Build history of the part. All positions in model axes, mm. Face numbers are marked on the shaded views. Give positions to 0.01 mm unless a question says otherwise; leave off trailing zeros. Order: outer loops, then holes, each group sorted by start corner. A loop starts at its lowest first (then second) coordinate and runs counter-clockwise, first axis right, second up. Notation, with made-up numbers: M -17.75,-26.5 L -13.75,-26.5 A15 ccw -13.75,1.5 Z; hole C 70.25,-22.5 d2. An arc over 180 degrees is marked long. Answer as CSV lines item,"result".
from build123d import *

# Parameters (mm, degrees)
CROQUIS1_W              = 120
CROQUIS1_H              = 120
CROQUIS1_R              = 3
CROQUIS1_W_2            = 80
CROQUIS1_H_2            = 80
SALIENTE_EXTRUIR1_DEPTH = 2.7


with BuildPart() as part:
    # Croquis1 → Saliente-Extruir1 (new body)
    with BuildSketch(Plane.XY):
        Rectangle(CROQUIS1_W, CROQUIS1_H)
        with Locations(Location((-40, 50, 0), (0, 0, 180))):
            Circle(CROQUIS1_R, mode=Mode.SUBTRACT)
        with Locations(Location((0, 50, 0), (0, 0, 180))):
            Circle(CROQUIS1_R, mode=Mode.SUBTRACT)
        with Locations(Location((40, 50, 0), (0, 0, 180))):
            Circle(CROQUIS1_R, mode=Mode.SUBTRACT)
        with Locations(Location((-40, -50, 0), (0, 0, 180))):
            Circle(CROQUIS1_R, mode=Mode.SUBTRACT)
        with Locations(Location((0, -50, 0), (0, 0, 180))):
            Circle(CROQUIS1_R, mode=Mode.SUBTRACT)
        with Locations(Location((40, -50, 0), (0, 0, 180))):
            Circle(CROQUIS1_R, mode=Mode.SUBTRACT)
        Rectangle(CROQUIS1_W_2, CROQUIS1_H_2, mode=Mode.SUBTRACT)
    extrude(amount=SALIENTE_EXTRUIR1_DEPTH)


solid = part.part
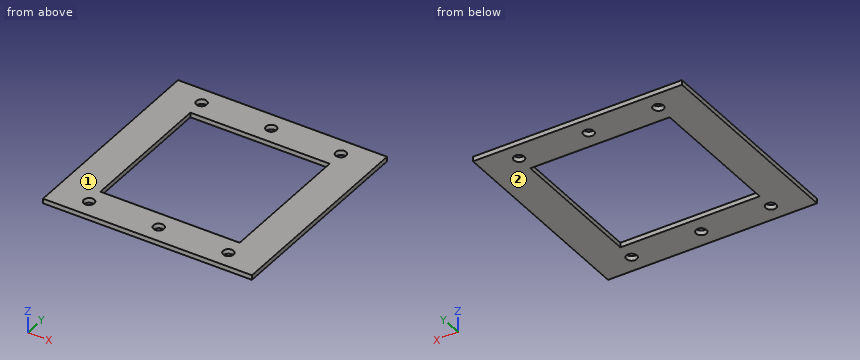
Item 1: Band-saw the part on A-A (x = -28.5). Give the cut face in (y, z), and give its area (3 significant figures).
Geometry says:
outline,"M -60,0 L -40,0 L -40,2.7 L -60,2.7 Z; M 40,0 L 60,0 L 60,2.7 L 40,2.7 Z"
area,"108 mm2"
Item 2: Band-saw the part on D-D (z = 1.85). Give the cut face in (x, y).
Geometry says:
outline,"M -60,-60 L 60,-60 L 60,60 L -60,60 Z; hole C -40,-50 d6; hole C -40,50 d6; hole M -40,-40 L 40,-40 L 40,40 L -40,40 Z; hole C 0,-50 d6; hole C 0,50 d6; hole C 40,-50 d6; hole C 40,50 d6"
Item 3: Band-saw the part on B-B (y = -50). Give the cut face in (x, z).
Geometry says:
outline,"M -60,0 L -43,0 L -43,2.7 L -60,2.7 Z; M -37,0 L -3,0 L -3,2.7 L -37,2.7 Z; M 3,0 L 37,0 L 37,2.7 L 3,2.7 Z; M 43,0 L 60,0 L 60,2.7 L 43,2.7 Z"
Item 4: Drop a flat-ended pin along its axis: pin 1 (7 mm diameter, centred on x = 40, y = 50, fed in from -Z). Give the stop position or say it passes through.
Geometry says:
pin 1,"stops at z = 0"
Item 5: Pull direction Z, two halves, no side cores. Call the marked faces 1 and 2: released by +Z, released by -Z, zero draft, split by the parting line, or undercut.
Geometry says:
face 1,"released by +Z"
face 2,"released by -Z"
Item 6: Probe line 1 along Y through (x, z) = (0, 1.8); line 2 along X through (y, z) = (50, 1.55); line 3 along X through (y, z) = (8, 1.8). List the from-to ranges inside material, lowest first. Write a range as from..to.
Geometry says:
line 1,"y = -60..-53, -47..-40, 40..47, 53..60"
line 2,"x = -60..-43, -37..-3, 3..37, 43..60"
line 3,"x = -60..-40, 40..60"
Item 7: Band-saw the part on C-C (x = 0). Give the cut face in (y, z).
Geometry says:
outline,"M -60,0 L -53,0 L -53,2.7 L -60,2.7 Z; M -47,0 L -40,0 L -40,2.7 L -47,2.7 Z; M 40,0 L 47,0 L 47,2.7 L 40,2.7 Z; M 53,0 L 60,0 L 60,2.7 L 53,2.7 Z"
